Drawing for the job (mm, zero at the part's lowest x, y, z). A direction names the side the tool comes from. Give positions to 0.01 mm unless a question says otherwise; leave off trailing zeros. Loops run counter-clockwise (first coordinate to the right, second up) from the corner with the lowest first, then second, coordinate; pieces in that order, holes last. Notation, with made-up numbers: M -20,44 L 35,44 A15 ccw 35,48 Z; hole C 27.25,40.25 d7. An arc over 180 degrees is marked long. Use CSV: the item, a comma, the result in double quotes. Start each with the question number.
(1) Slice it at B-B on x = 18. List the corners of the cut face in (y, z), and give its area (3 significant figures).
(2) Two-plate mould, pull along X, no slides. Class the marked faces 1, 2 and 3: pulls with the +X half, pulls with the -X half, needs draft (parallel to the pull), parting line crosses it, or undercut.
(3) Tool access for the marked faces 4, 5 and 6: list every direction of +Z, -Z, +X, -X, +Y, -Y with a clear straight run to the whole face (end or side of a thin tool).
(4) Wall check: line 1 along Y through (x, z) = (10.9, 3.6) (3 decimals); line 2 along Y through (x, z) = (10.9, 5.5); line 3 along Y through (x, z) = (3.4, 2.65). Give the ranges that are in metal, low to high. Write a range as from..to.
(5) Slice it at C-C on z = 10.5. List the corners of the cut face in (x, y), and give its area (3 significant figures).
(6) Flat gauge pins, fed straight in: P1, Ø6, axis at y = 5, z = 9.5, coming from the -X side; P2, Ø1, axis at y = 6, z = 3, coming from the +X side; P3, Ø1, axis at x = 15.5, z = 4.5, coming from the -Y side. Where does each tip first touch, or does it go through?
(7) Slice it at D-D on z = 3. List the corners of the cut face in (x, y) (3 decimals).
(8) Slice it at A-A on y = 10.9. List the corners of the cut face in (x, z), and give its area (3 significant figures).
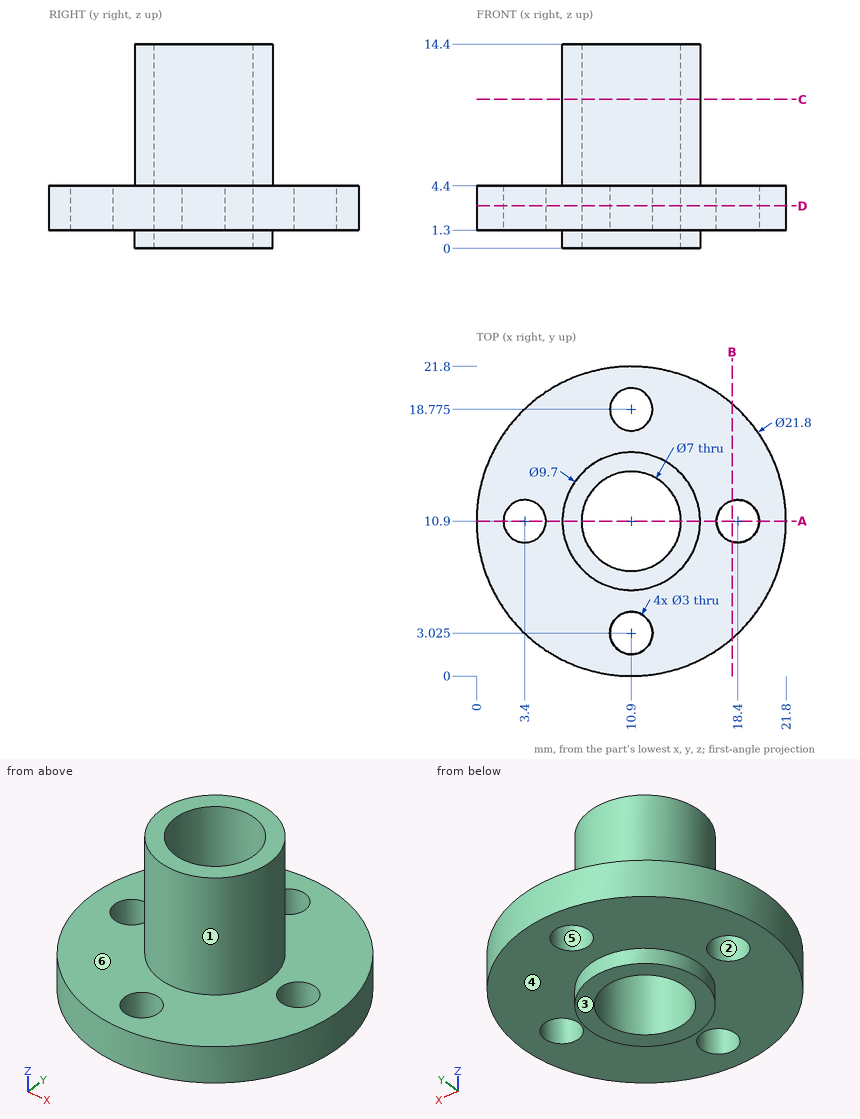
Reply:
1,outline,"M 2.63,1.3 L 9.45,1.3 L 9.45,4.4 L 2.63,4.4 Z; M 12.35,1.3 L 19.17,1.3 L 19.17,4.4 L 12.35,4.4 Z"
1,area,"42.3 mm^2"
2,face 1,"parting line crosses it"
2,face 2,"undercut"
2,face 3,"needs draft"
3,face 4,"-Z"
3,face 5,"+Z, -Z"
3,face 6,"+Z"
4,line 1,"y = 0..1.525, 4.525..7.4, 14.4..17.275, 20.275..21.8"
4,line 2,"y = 6.05..7.4, 14.4..15.75"
4,line 3,"y = 2.99..9.4, 12.4..18.81"
5,outline,"C 10.9,10.9 d9.7; hole C 10.9,10.9 d7"
5,area,"35.4 mm^2"
6,P1,"stops at x = 7.01"
6,P2,"stops at x = 20.87"
6,P3,"stops at y = 0.8"
7,outline,"C 10.9,10.9 d21.8; hole C 3.4,10.9 d3; hole C 10.9,10.9 d7; hole C 10.9,3.025 d3; hole C 10.9,18.775 d3; hole C 18.4,10.9 d3"
8,outline,"M 0,1.3 L 1.9,1.3 L 1.9,4.4 L 0,4.4 Z; M 4.9,1.3 L 6.05,1.3 L 6.05,0 L 7.4,0 L 7.4,14.4 L 6.05,14.4 L 6.05,4.4 L 4.9,4.4 Z; M 14.4,0 L 15.75,0 L 15.75,1.3 L 16.9,1.3 L 16.9,4.4 L 15.75,4.4 L 15.75,14.4 L 14.4,14.4 Z; M 19.9,1.3 L 21.8,1.3 L 21.8,4.4 L 19.9,4.4 Z"
8,area,"57.8 mm^2"
